from build123d import *

# Parameters (mm, degrees)
SKETCH1_W            = 31.8
SKETCH1_H            = 3.2
BOSS_EXTRUDE1_DEPTH  = 15.8
SKETCH2_R            = 2.4
BOSS_EXTRUDE2_DEPTH  = 1.6
LPATTERN1_COUNT      = 2
LPATTERN1_PITCH      = 8
LPATTERN1_COUNT_DIR2 = 6
LPATTERN1_PITCH_DIR2 = 8
SHELL1_T             = -1.2
SKETCH3_R            = 3.25
SKETCH3_R_2          = 2.4
BOSS_EXTRUDE3_DEPTH  = 1.8
SKETCH4_W            = 0.8
SKETCH4_H            = 13.4
BOSS_EXTRUDE4_DEPTH  = 1.8
BOSS_EXTRUDE5_DEPTH  = 1.2
SKETCH7_R            = 2.95
BOSS_EXTRUDE6_DEPTH  = 1
SKETCH8_R            = 2.2
SKETCH8_R_2          = 1.5
BOSS_EXTRUDE7_DEPTH  = 7.7
BOSS_EXTRUDE8_START  = -0.5
SKETCH9_R            = 2.5
SKETCH9_R_2          = 2.2
BOSS_EXTRUDE8_DEPTH  = 0.5
CUT_EXTRUDE1_START   = -3.7
CUT_EXTRUDE1_DEPTH   = 3.7


with BuildPart() as part:
    # Sketch1 → Boss-Extrude1 (new body)
    with BuildSketch(Plane.XY):
        with Locations((15.9, 1.6)):
            Rectangle(SKETCH1_W, SKETCH1_H)
    extrude(amount=-BOSS_EXTRUDE1_DEPTH)

    # Sketch2 → Boss-Extrude2 (add)
    with BuildSketch(Plane(origin=(0, 3.2, 0), x_dir=(1, 0, 0), z_dir=(0, 1, 0))):
        with Locations(Location((3.9, 3.9, 0), (0, 0, 270))):
            Circle(SKETCH2_R)
    boss_extrude2 = extrude(amount=BOSS_EXTRUDE2_DEPTH)

    # LPattern1: Boss-Extrude2 2 × 6, 4 skipped
    with Locations(*[(j * LPATTERN1_PITCH_DIR2, 0, -i * LPATTERN1_PITCH) for i in range(LPATTERN1_COUNT) for j in range(LPATTERN1_COUNT_DIR2) if (i, j) not in ((0, 0), (0, 4), (0, 5), (1, 4), (1, 5))]):
        add(boss_extrude2)

    # Shell1
    shell1_openings = [part.faces().sort_by_distance(p)[0] for p in [
        (15.9, 0, -7.9),
    ]]
    offset(amount=SHELL1_T, openings=shell1_openings, kind=Kind.INTERSECTION)

    # Sketch3 → Boss-Extrude3 (add)
    with BuildSketch(Plane.XZ.offset(-2)):
        with Locations(Location((15.9, -7.9, 0), (0, 0, 90))):
            Circle(SKETCH3_R)
        with Locations(Location((15.9, -7.9, 0), (0, 0, 270))):
            Circle(SKETCH3_R_2, mode=Mode.SUBTRACT)
    extrude(amount=BOSS_EXTRUDE3_DEPTH)

    # Sketch4 → Boss-Extrude4 (add)
    with BuildSketch(Plane.XZ.offset(-2)):
        with Locations((9.1, -7.9)):
            Rectangle(SKETCH4_W, SKETCH4_H)
        with Locations((22.7, -7.9)):
            Rectangle(SKETCH4_W, SKETCH4_H)
    extrude(amount=BOSS_EXTRUDE4_DEPTH)

    # Sketch5 → Boss-Extrude5 (add)
    with BuildSketch(Plane(origin=(31.8, 0, 0), x_dir=(0, 0, -1), z_dir=(1, 0, 0))):
        Polygon((6.3, -3.2), (9.5, -3.2), (12.5, 0), (3.3, 0), align=None)
    boss_extrude5 = extrude(amount=-BOSS_EXTRUDE5_DEPTH)

    # Mirror1: Boss-Extrude5 across plane
    add(boss_extrude5.mirror(Plane.ZY.offset(-15.9)))

    # Sketch7 → Boss-Extrude6 (add)
    with BuildSketch(Plane(origin=(31.8, 0, 0), x_dir=(0, 0, -1), z_dir=(1, 0, 0))):
        with Locations(Location((7.9, -0.25, 0), (0, 0, 270))):
            Circle(SKETCH7_R)
    boss_extrude6 = extrude(amount=BOSS_EXTRUDE6_DEPTH)

    # Sketch8 → Boss-Extrude7 (add)
    with BuildSketch(Plane(origin=(32.8, 0, 0), x_dir=(0, 0, -1), z_dir=(1, 0, 0))):
        with Locations(Location((7.9, -0.25, 0), (0, 0, 180))):
            Circle(SKETCH8_R)
        with Locations(Location((7.9, -0.25, 0), (0, 0, 180))):
            Circle(SKETCH8_R_2, mode=Mode.SUBTRACT)
    boss_extrude7 = extrude(amount=BOSS_EXTRUDE7_DEPTH)

    # Sketch9 → Boss-Extrude8 (add)
    with BuildSketch(Plane(origin=(40.5, 0, 0), x_dir=(0, 0, -1), z_dir=(1, 0, 0)).offset(BOSS_EXTRUDE8_START)):
        with Locations((7.9, -0.25)):
            Circle(SKETCH9_R)
        with Locations(Location((7.9, -0.25, 0), (0, 0, 180))):
            Circle(SKETCH9_R_2, mode=Mode.SUBTRACT)
    boss_extrude8 = extrude(amount=BOSS_EXTRUDE8_DEPTH)

    # Sketch10 → Cut-Extrude1 (cut)
    with BuildSketch(Plane(origin=(40.5, 0, 0), x_dir=(0, 0, -1), z_dir=(1, 0, 0)).offset(CUT_EXTRUDE1_START)):
        with BuildLine():
            Line((7.9, -1.75), (7.9, -2.75))
            ThreePointArc((7.9, -2.75), (8.151272405, -2.737340383), (8.4, -2.699489743))
            Line((8.4, -2.699489743), (8.4, -1.664213562))
            ThreePointArc((8.4, -1.664213562), (8.153652968, -1.728397839), (7.9, -1.75))
        make_face()
        with BuildLine():
            Line((7.9, 2.25), (7.9, 1.25))
            ThreePointArc((7.9, 1.25), (8.153652968, 1.228397839), (8.4, 1.164213562))
            Line((8.4, 1.164213562), (8.4, 2.199489743))
            ThreePointArc((8.4, 2.199489743), (8.151272405, 2.237340383), (7.9, 2.25))
        make_face()
        with BuildLine():
            ThreePointArc((7.4, -2.699489743), (7.648727595, -2.737340383), (7.9, -2.75))
            Line((7.9, -2.75), (7.9, -1.75))
            ThreePointArc((7.9, -1.75), (7.646347032, -1.728397839), (7.4, -1.664213562))
            Line((7.4, -1.664213562), (7.4, -2.699489743))
        make_face()
        with BuildLine():
            ThreePointArc((7.4, 1.164213562), (7.646347032, 1.228397839), (7.9, 1.25))
            Line((7.9, 1.25), (7.9, 2.25))
            ThreePointArc((7.9, 2.25), (7.648727595, 2.237340383), (7.4, 2.199489743))
            Line((7.4, 2.199489743), (7.4, 1.164213562))
        make_face()
    cut_extrude1 = extrude(amount=CUT_EXTRUDE1_DEPTH, mode=Mode.SUBTRACT)

    # Mirror2: Boss-Extrude6, Boss-Extrude7, Boss-Extrude8, Cut-Extrude1 across plane
    add(boss_extrude6.mirror(Plane.ZY.offset(-15.9)))
    add(boss_extrude7.mirror(Plane.ZY.offset(-15.9)))
    add(boss_extrude8.mirror(Plane.ZY.offset(-15.9)))
    add(cut_extrude1.mirror(Plane.ZY.offset(-15.9)), mode=Mode.SUBTRACT)


solid = part.part
Design review of the part built by this model. Coordinates are the model's own, in mm. A direction names the side the tool comes from. Round coordinates to 2 decimals unless told otherwise and drop trailing zeros. Loops run counter-clockwise (first coordinate to the right, second up) from the corner with the lowest first, then second, coordinate; pieces in that order, holes last. Notation, with made-up numbers: (19.5, -38.75) - (61.5, -38.75) arc R16 ccw to (61.5, -19.75) - close; hole circle Ø1 at (50, -23). An arc over 180 degrees is marked (long way). One line per question, with ' | ' between items.
1. We need section B-B, the plane x = -2. State the section outline as (y, z) points, and give its area (3 significant figures).
Results are:
outline: circle Ø4.4 at (-0.25, -7.9); hole circle Ø3 at (-0.25, -7.9) | area: 8.14 mm²
2. For faces 1 (the face through (32.8, 0, -8)), 2 (the face through (-1, 2, -7)), 3 (the face through (5, 2, -8)), list the 3-axis set-ups (+Z, -Z, +X, -X, +Y, -Y) from which the entire face can be reached by the end or side of a thin tool; tool diameter is ignored.
Results are:
face 1: +X | face 2: none | face 3: -Y
3. Draft analysis for pull direction Z (two halves, no side actions). For faces 4 (the face through (12, 4.8, -4)), 5 (the face through (9, 0.2, -8)), 6 (the face through (25.557, 3.989, -12.42)), 7 (the face through (-8.4, -0.2, -5.4)), state which applies: released by +Z, released by -Z, zero draft, split by the parting line, or undercut.
Results are:
face 4: zero draft | face 5: undercut | face 6: undercut | face 7: released by +Z
4. Clearance check with flat-ended pins moving along their axes: P1, Ø0.7, axis at x = 19.5, z = -3.5, coming from the -Y side; P2, Ø1, axis at y = 0, z = -2.5, coming from the +X side; P3, Ø4, axis at x = 18.5, z = -7.5, coming from the -Y side; P4, Ø3, axis at y = 0, z = -9, coming from the +X side. State where each tip first meets the part, or that it passes through.
Results are:
P1: stops at y = 3.6 | P2: stops at x = 31.8 | P3: stops at y = 0.2 | P4: stops at x = 40.5
5. We need section A-A, the plane x = 27.9. State the section outline as (y, z) points, and give its area (3 significant figures).
Results are:
outline: (0, -15.8) - (3.2, -15.8) - (3.2, -14.3) - (4.8, -14.3) - (4.8, -9.5) - (3.2, -9.5) - (3.2, -6.3) - (4.8, -6.3) - (4.8, -1.5) - (3.2, -1.5) - (3.2, 0) - (0, 0) - (0, -1.2) - (2, -1.2) - (2, -2.7) - (3.6, -2.7) - (3.6, -5.1) - (2, -5.1) - (2, -10.7) - (3.6, -10.7) - (3.6, -13.1) - (2, -13.1) - (2, -14.6) - (0, -14.6) - close | area: 31.4 mm²
6. For L1, parallel to X at y = 3.05, z = -11.9; L2, parallel to X at y = 1.75, z = -4; L3, parallel to Z at x = 11.9, y = 2.9, list the stretches that pass through material, from the lowest coordinate up. Write a range as [from, to].
Results are:
L1: x = [0, 2.7], [5.1, 10.7], [13.1, 18.7], [21.1, 26.7], [29.1, 31.8] | L2: x = [0, 1.2], [8.7, 9.5], [22.3, 23.1], [30.6, 31.8] | L3: z = [-15.8, -13.1], [-10.7, -5.1], [-2.7, 0]
